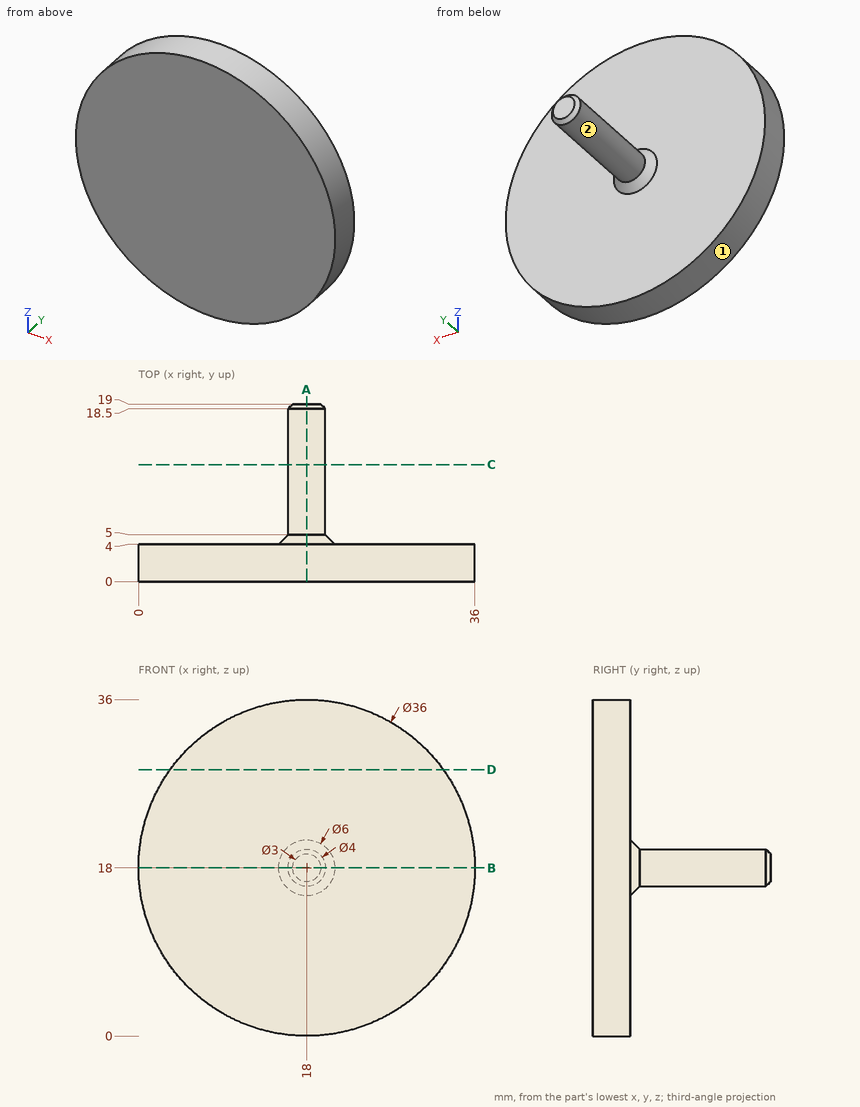
The figure shows three views and two pictorial views of one solid part (mm, origin at its lowest corner). Answer the questions. A direction names the side the tool comes from. Give positions to 0.01 mm unless a question says otherwise; leave off trailing zeros. Order: outer loops, then holes, each group sorted by start corner. A loop starts at its lowest first (then second) coordinate and runs counter-clockwise, first axis right, second up. Notation, with made-up numbers: (-36.5, 8) -> (-30.5, 8) arc R32 ccw to (-30.5, 34) -> close; hole circle Ø10 at (-34, 40.5). An arc over 180 degrees is marked (long way). Answer as CSV lines item,"result". Start each with the question number.
Q1. Given pin 1 (3 mm diameter, centred on x = 4, z = 31, fed in from +Y); pin 2 (8 mm diameter, centred on x = 15.5, y = 5, fed in from +Z); pin 3 (5 mm diameter, centred on x = 17, z = 19, fed in from -Y), each flat-ended and moving along its own axis, determine where each tip first touches the part or whether it passes through.
Q2. Find the intervals of material crossed by L1, parallel to Y at x = 23, z = 10; L2, parallel to Z at x = 11, y = 3.25; L3, parallel to Z at x = 4, y = 1.75, in increasing order.
Q3. A cutting plane is placed at D-D (z = 28.5). Determine the outline of the cut face in (x, y).
Q4. A cutting plane is placed at B-B (z = 18). Determine the outline of the cut face in (x, y).
Q5. A cutting plane is placed at C-C (y = 12.5). Determine the outline of the cut face in (x, z), then the cut area to 3 significant figures.
Q6. Which of the six approach directions +Z, -Z, +X, -X, +Y, -Y give full straight-line access (tool end or side, diameter ignored) to the marked faces 1 and 2?
Q7. A cutting plane is placed at A-A (x = 18). Determine the outline of the cut face in (y, z).
Results found:
1,pin 1,"y = 4"
1,pin 2,"z = 36"
1,pin 3,"y = 0"
2,L1,"0 to 4"
2,L2,"1.42 to 34.58"
2,L3,"6.69 to 29.31"
3,outline,"(3.38, 0) -> (32.62, 0) -> (32.62, 4) -> (3.38, 4) -> close"
4,outline,"(0, 0) -> (36, 0) -> (36, 4) -> (21, 4) -> (20, 5) -> (20, 18.5) -> (19.5, 19) -> (16.5, 19) -> (16, 18.5) -> (16, 5) -> (15, 4) -> (0, 4) -> close"
5,outline,"circle Ø4 at (18, 18)"
5,area,"12.6 mm2"
6,face 1,"+Y, -Y"
6,face 2,"+Y"
7,outline,"(0, 0) -> (4, 0) -> (4, 15) -> (5, 16) -> (18.5, 16) -> (19, 16.5) -> (19, 19.5) -> (18.5, 20) -> (5, 20) -> (4, 21) -> (4, 36) -> (0, 36) -> close"
